Verification items for this drawing (mm, ordinates from the low corner). Round coordinates to 2 decimals unless told otherwise and drop trailing zeros. Order: outer loops, then holes, each group sorted by start corner. A loop starts at its lowest first (then second) coordinate and runs counter-clockwise, first axis right, second up. Notation, with made-up numbers: M 84.25,-10.5 L 130.25,-10.5 A20 cw 130.25,1.5 Z; hole C 54.5,86.5 d10. An arc over 180 degrees is marked long. Return JSON: item names as keys, results as strings. Group by question number.
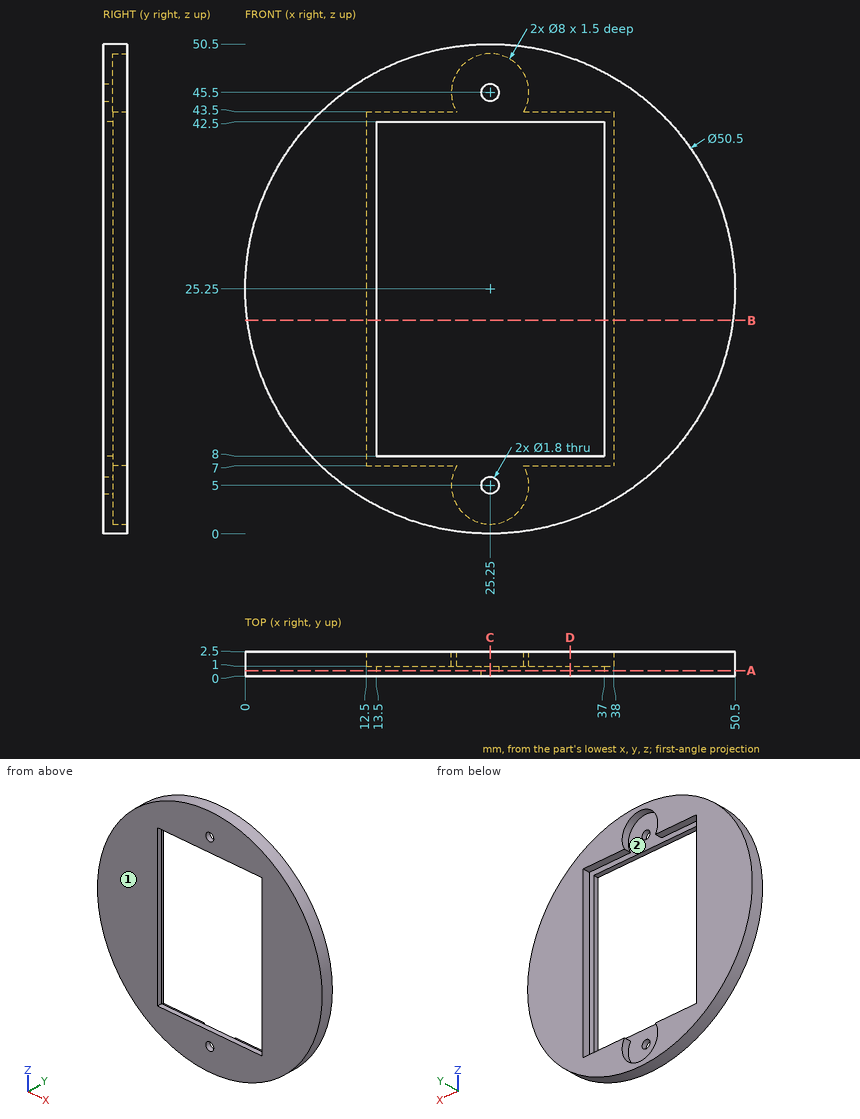
Q1. Section check C-C on x = 25.25. Record the cut outline in (y, z), plus the area to 3 significant figures.
Q2. Release check for a two-part mould opening along X. For the marked faces 1 and 2 record: +X half, -X half, draft (parallel to the pull), parting line (faces both ways), or undercut.
Q3. Depth check by flat-ended pin: pin 1 Ø0.8 at (y, z) = (1.5, 23.5) entering from +X; pin 2 Ø1.1 at (y, z) = (0.5, 29) entering from -X; pin 3 Ø1 at (x, y) = (16.5, 2) entering from -Z. Enter the tip coordinate at first touch or a pass-through.
Q4. Section check B-B on z = 22. Record the cut outline in (x, y), plus the area to 4 significant figures.
Q5. Section check D-D on x = 33.5. Record the cut outline in (y, z).
Q6. Section check A-A on y = 0.55. Record the cut outline in (x, z).
Q7. Material ranges on line 1 along Z through (x, y) = (25.25, 0.35); line 2 along Z through (x, y) = (15, 1.95); line 3 along X through (y, z) = (0.5, 26.5), recorded low to high.
Geometry check:
{
 "1": {"outline": "M 0,0 L 2.5,0 L 2.5,1 L 1,1 L 1,4.1 L 0,4.1 Z; M 0,5.9 L 1,5.9 L 1,8 L 0,8 Z; M 0,42.5 L 1,42.5 L 1,44.6 L 0,44.6 Z; M 0,46.4 L 1,46.4 L 1,49.5 L 2.5,49.5 L 2.5,50.5 L 0,50.5 Z", "area": "15.4 mm^2"},
 "2": {"face 1": "draft", "face 2": "undercut"},
 "3": {"pin 1": "stops at x = 50.46", "pin 2": "stops at x = 0.2", "pin 3": "stops at z = 1.39"},
 "4": {"outline": "M 0.21,0 L 13.5,0 L 13.5,1 L 12.5,1 L 12.5,2.5 L 0.21,2.5 Z; M 37,0 L 50.29,0 L 50.29,2.5 L 38,2.5 L 38,1 L 37,1 Z", "area": "63.45 mm^2"},
 "5": {"outline": "M 0,1.39 L 2.5,1.39 L 2.5,7 L 1,7 L 1,8 L 0,8 Z; M 0,42.5 L 1,42.5 L 1,43.5 L 2.5,43.5 L 2.5,49.11 L 0,49.11 Z"},
 "6": {"outline": "C 25.25,25.25 d50.5; hole M 13.5,8 L 37,8 L 37,42.5 L 13.5,42.5 Z; hole C 25.25,5 d1.8; hole C 25.25,45.5 d1.8"},
 "7": {"line 1": "z = 0 to 4.1, 5.9 to 8, 42.5 to 44.6, 46.4 to 50.5", "line 2": "z = 2.17 to 7, 43.5 to 48.33", "line 3": "x = 0.03 to 13.5, 37 to 50.47"}
}
